Autodesk Inventor part; units mm, degrees
ref_plane "YZ Plane" through (0, 0, 0) normal (1, 0, 0) x (0, 1, 0)
ref_plane "XZ Plane" through (0, 0, 0) normal (0, 1, 0) x (-1, 0, 0)
ref_plane "XY Plane" through (0, 0, 0) normal (0, 0, 1) x (1, 0, 0)
sketch "Sketch1" plane through (0, 0, 0) normal (0, 1, 0) x (-1, 0, 0)
  circle A0 centre (0, 0) radius 12
  dimension "d0" = 24
extrude "Extrusion1" add sketch "Sketch1" along normal blind 2
sketch "Sketch2" plane through (0, 2, 0) normal (0, 1, 0) x (1, 0, 0)
  circle A0 centre (0, 0) radius 4
  dimension "d3" = 8
extrude "Extrusion2" add sketch "Sketch2" along normal blind 3
sketch "Sketch3" plane through (0, 5, 0) normal (0, 1, 0) x (1, 0, 0)
  point P0 (0, 0)
  point P1 (0, 0)
hole "Hole1" at (0, 5, 0) direction (0, -1, 0) diameter 3 end through all counterbore diameter 4 counterbore depth 1
sketch "Sketch4" plane through (0, 2, 0) normal (0, 1, 0) x (1, 0, 0)
  circle A0 centre (-9.25, 0) radius 0.5
  line L0 (0, 0) -> (-9.25, 0) construction
  line L1 (0, 0) -> (-9.1094, 2.4408) construction
  line L2 (0, 0) -> (-9.1094, -2.4408) construction
  circle A1 centre (-9.1094, 2.4408) radius 0.5
  circle A2 centre (-9.1094, -2.4408) radius 0.5
  circle A3 centre (0, 0) radius 12
  circle A4 centre (12, 0) radius 21.25 construction
  dimension "d13" = 15
  dimension "d14" = 15
  dimension "d15" = 1
  dimension "d16" = 1
  dimension "d17" = 1
  dimension "d25" = 9.25
extrude "Extrusion3" cut sketch "Sketch4" against normal through all contours A0 | A1 | A2
pattern_circular "Circular Pattern1" count 4 over 360 about axis through (0, -29.8074, 0) along (0, 1, 0) of "Extrusion3"
properties part number "Servo wheel"
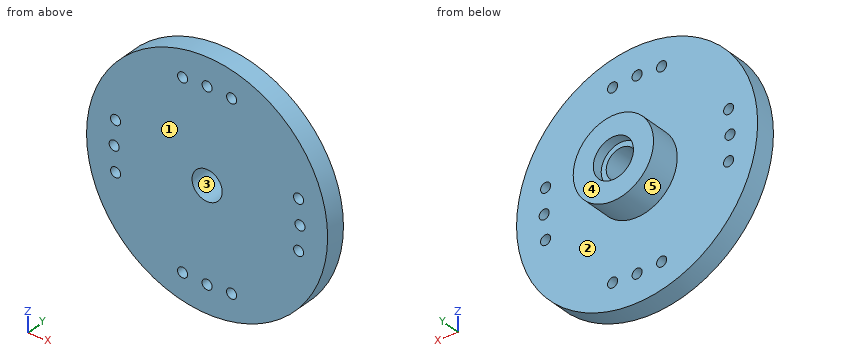
Verification items for the finished model (mm, model axes). Face numbers are marked on the shaded views. A direction names the side the tool comes from. Coordinates: 2 decimals unless noted, no trailing zeros. Loops run counter-clockwise (first coordinate to the right, second up) from the corner with the lowest first, then second, coordinate; pieces in that order, holes last. Notation, with made-up numbers: (18, 27) - (70, 27) arc R21 cw to (70, 41) - close; hole circle Ø9 at (76.5, 64). An arc over 180 degrees is marked (long way). Answer as a JSON object with one key per item and string values.
(1) Cross-section at D-D, the plane x = 9.25. Record the boundary of the cut face in (y, z), then the cut area to 3 significant figures.
Response:
{"outline": "(0, -7.64) - (2, -7.64) - (2, -2.92) - (0, -2.92) - close; (0, -1.96) - (2, -1.96) - (2, -0.5) - (0, -0.5) - close; (0, 0.5) - (2, 0.5) - (2, 1.96) - (0, 1.96) - close; (0, 2.92) - (2, 2.92) - (2, 7.64) - (0, 7.64) - close", "area": "24.7 mm²"}
(2) Cross-section at B-B, the plane y = 2.85. Record the boundary of the cut face in (x, z), then the cut area to 3 significant figures.
Response:
{"outline": "circle Ø8 at (0, 0); hole circle Ø3 at (0, 0)", "area": "43.2 mm²"}
(3) Go/stop test with flat-tipped pins: pin 1 Ø2 at (x, y) = (-3.5, 1) entering from -Z; pin 2 Ø3 at (y, z) = (3, 3.5) entering from -X; pin 3 Ø6 at (x, z) = (-0.5, 9) entering from +Y. Record where each tip stops, or that it passes through.
Response:
{"pin 1": "stops at z = -11.74", "pin 2": "stops at x = -11.76", "pin 3": "stops at y = 2"}
(4) Access from +Z, -Z, +X, -X, +Y, -Y to the whole of each face (thin tool, end or side, straight path). Record for the marked faces 1 and 2.
Response:
{"face 1": "+Z, -Z, +X, -X, -Y", "face 2": "+Y"}
(5) Cross-section at A-A, the plane x = 0. Record the boundary of the cut face in (y, z).
Response:
{"outline": "(0, -12) - (2, -12) - (2, -9.75) - (0, -9.75) - close; (0, -8.75) - (2, -8.75) - (2, -4) - (5, -4) - (5, -2) - (4, -2) - (4, -1.5) - (0, -1.5) - close; (0, 1.5) - (4, 1.5) - (4, 2) - (5, 2) - (5, 4) - (2, 4) - (2, 8.75) - (0, 8.75) - close; (0, 9.75) - (2, 9.75) - (2, 12) - (0, 12) - close"}
(6) Scan lines: line 1 along X through (y, z) = (3.1, 0); line 2 along Z through (x, y) = (2.25, 1.9). Record each from-to range of solid material in increasing order.
Response:
{"line 1": "x = -4 to -1.5, 1.5 to 4", "line 2": "z = -11.79 to -9.57, -8.65 to 8.65, 9.57 to 11.79"}
(7) Mould release check, pull along Z, two halves, no side actions. Record for the marked faces 3, 4 and 5: pulls with the +Z half, pulls with the -Z half, needs draft (parallel to the pull), parting line crosses it, or undercut.
Response:
{"face 3": "undercut", "face 4": "needs draft", "face 5": "parting line crosses it"}
(8) Cross-section at C-C, the plane y = 0.4. Count the separate pieces of the cut face and the enclosed holes in it, then the cut area to 3 significant figures.
Response:
{"separate pieces": "1", "enclosed holes": "13", "area": "436 mm²"}
